Geometry: final body of the model. Coordinates: model frame, mm. Face numbers are marked on the shaded views. Give positions to 0.01 mm unless a question says otherwise; leave off trailing zeros. Use one line per item in the form item = value. Start each with the question number.
Item 1: Material intervals for line 1 along X through (y, z) = (-100, 479); line 2 along X through (y, z) = (734, 250); line 3 along Z through (x, y) = (15, 410), sorted ascending. Write a range as from..to.
Item 2: Contact query for flat-ended pins moving along their axis: P1, Ø16, axis at x = 25, z = 350, coming from the -Y side; P2, Ø8.5, axis at x = 25, z = 450, coming from the +Y side; P3, Ø12, axis at x = 25, y = 300, coming from the +Z side; P4, Ø11, axis at x = 25, z = -450, coming from the +Y side. Output: stop coordinate, or through.
Item 3: Pull-direction query (X, two-part tool) for the marked faces 1 and 2; classes: released by +X, released by -X, zero draft, split by the parting line, or undercut.
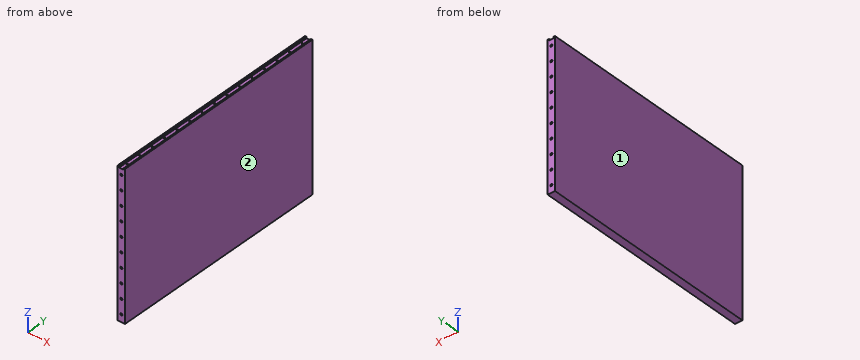
from build123d import *

# Parameters (mm, degrees)
F0_W     = 1500
F0_H     = 1000
F1_DEPTH = 50
F3_D     = 10.3
F3_DEPTH = 25.25
F3_TIP   = 3.094432188
F4_W     = 30
F4_H     = 10
F5_DEPTH = 1500.001
F7_D     = 14
F7_DEPTH = 31
F7_TIP   = 4.2060243332
F9_D     = 14
F9_DEPTH = 31
F9_TIP   = 4.2060243332


with BuildPart() as f1:
    # F0 (on Right) → F1 (new body)
    with BuildSketch(Plane.YZ):
        Rectangle(F0_W, F0_H)
    extrude(amount=F1_DEPTH)

    # F3
    with Locations(Plane.XY.offset(500)):
        with Locations((25, -700), (25, -600), (25, -500), (25, -400), (25, -300), (25, -200), (25, -100), (25, 0), (25, 200), (25, 100), (25, 300), (25, 400), (25, 500), (25, 700), (25, 600)):
            Hole(F3_D / 2, depth=F3_DEPTH)
            with Locations((0, 0, -(F3_DEPTH + F3_TIP / 2))):  # 118° drill point
                Cone(0, F3_D / 2, F3_TIP, mode=Mode.SUBTRACT)

    # F4 (on face) → F5 (cut, through all)
    with BuildSketch(Plane.XZ.offset(750)):
        with Locations((25, 495)):
            Rectangle(F4_W, F4_H)
    extrude(amount=-F5_DEPTH, mode=Mode.SUBTRACT)

    # F7
    with Locations(Plane.XZ.offset(750)):
        with Locations((25, -450), (25, -350), (25, -250), (25, -150), (25, -50), (25, 50), (25, 450), (25, 350), (25, 250), (25, 150)):
            Hole(F7_D / 2, depth=F7_DEPTH)
            with Locations((0, 0, -(F7_DEPTH + F7_TIP / 2))):  # 118° drill point
                Cone(0, F7_D / 2, F7_TIP, mode=Mode.SUBTRACT)

    # F9
    with Locations(Plane(origin=(0, 750, 0), x_dir=(-1, 0, 0), z_dir=(0, 1, 0))):
        with Locations((-25, 450), (-25, 350), (-25, 250), (-25, 150), (-25, 50), (-25, -50), (-25, -150), (-25, -250), (-25, -350), (-25, -450)):
            Hole(F9_D / 2, depth=F9_DEPTH)
            with Locations((0, 0, -(F9_DEPTH + F9_TIP / 2))):  # 118° drill point
                Cone(0, F9_D / 2, F9_TIP, mode=Mode.SUBTRACT)


solid = f1.part
Answer sheet:
q1.line_1 = 0..19.85, 30.15..50
q1.line_2 = 0..18, 32..50
q1.line_3 = -500..490
q2.P1 = -750
q2.P2 = 717.35
q2.P3 = 490
q2.P4 = 718.1
q3.face_1 = released by -X
q3.face_2 = released by +X
